from build123d import *

# Parameters (mm, degrees)
SKETCH2_R                           = 26
BOSS_EXTRUDE1_DEPTH                 = 110
CUT_EXTRUDE1_REACH                  = 117.983
CUT_EXTRUDE1_END_RADIUS             = 26
SKETCH3_W                           = 35
SKETCH3_H                           = 25
CUT_EXTRUDE1_DIRECTION_2_REACH      = 117.983
CUT_EXTRUDE1_DIRECTION_2_END_RADIUS = 26
CUT_EXTRUDE2_REACH                  = 118.211
CUT_EXTRUDE2_END_RADIUS             = 26
SKETCH4_R                           = 6
CUT_EXTRUDE4_REACH                  = 117.983
SKETCH6_W                           = 22
SKETCH6_H                           = 16
CUT_EXTRUDE4_DIRECTION_2_REACH      = 117.983


with BuildPart() as part:
    # Sketch2 → Boss-Extrude1 (new body)
    with BuildSketch(Plane(origin=(0, 0, 0), x_dir=(0, 0, -1), z_dir=(1, 0, 0))):
        Circle(SKETCH2_R)
    extrude(amount=BOSS_EXTRUDE1_DEPTH)

    # Cut-Extrude1: up to this cylinder (the profile starts inside it)
    cut_extrude1_end = Plane(origin=(54.2237205, 0, 0), z_dir=(-1, 0, 0)) * Cylinder(CUT_EXTRUDE1_END_RADIUS, 362.413441, mode=Mode.PRIVATE)
    # Sketch3 → Cut-Extrude1 (cut, up to the surface)
    with BuildSketch(Plane.XY, mode=Mode.PRIVATE) as cut_extrude1_sk1:
        with Locations((17.5, 13.5)):
            Rectangle(SKETCH3_W, SKETCH3_H)
    cut_extrude1_tool1 = extrude(cut_extrude1_sk1.sketch, amount=-CUT_EXTRUDE1_REACH, mode=Mode.PRIVATE) & cut_extrude1_end
    add(cut_extrude1_tool1.solids().sort_by_distance((17.5, 13.5, 0))[0], mode=Mode.SUBTRACT)
    # Sketch3 → Cut-Extrude1 (cut, up to the surface)
    with BuildSketch(Plane.XY, mode=Mode.PRIVATE) as cut_extrude1_sk2:
        Polygon((52.84232335, 26), (110, -7), (110, 26), align=None)
    cut_extrude1_tool2 = extrude(cut_extrude1_sk2.sketch, amount=-CUT_EXTRUDE1_REACH, mode=Mode.PRIVATE) & cut_extrude1_end
    add(cut_extrude1_tool2.solids().sort_by_distance((90.947441, 15, 0))[0], mode=Mode.SUBTRACT)

    # Cut-Extrude1 direction 2: up to this cylinder (the profile starts inside it)
    cut_extrude1_direction_2_end = Plane(origin=(54.2237205, 0, 0), z_dir=(-1, 0, 0)) * Cylinder(CUT_EXTRUDE1_DIRECTION_2_END_RADIUS, 362.413441, mode=Mode.PRIVATE)
    # Sketch3 → Cut-Extrude1 direction 2 (cut, up to the surface)
    with BuildSketch(Plane.XY, mode=Mode.PRIVATE) as cut_extrude1_direction_2_sk1:
        with Locations((17.5, 13.5)):
            Rectangle(SKETCH3_W, SKETCH3_H)
    cut_extrude1_direction_2_tool1 = extrude(cut_extrude1_direction_2_sk1.sketch, amount=CUT_EXTRUDE1_DIRECTION_2_REACH, mode=Mode.PRIVATE) & cut_extrude1_direction_2_end
    add(cut_extrude1_direction_2_tool1.solids().sort_by_distance((17.5, 13.5, 0))[0], mode=Mode.SUBTRACT)
    # Sketch3 → Cut-Extrude1 direction 2 (cut, up to the surface)
    with BuildSketch(Plane.XY, mode=Mode.PRIVATE) as cut_extrude1_direction_2_sk2:
        Polygon((52.84232335, 26), (110, -7), (110, 26), align=None)
    cut_extrude1_direction_2_tool2 = extrude(cut_extrude1_direction_2_sk2.sketch, amount=CUT_EXTRUDE1_DIRECTION_2_REACH, mode=Mode.PRIVATE) & cut_extrude1_direction_2_end
    add(cut_extrude1_direction_2_tool2.solids().sort_by_distance((90.947441, 15, 0))[0], mode=Mode.SUBTRACT)

    # Cut-Extrude2: up to this cylinder (the profile starts inside it)
    cut_extrude2_end = Plane(origin=(12, 0, 0), z_dir=(-1, 0, 0)) * Cylinder(CUT_EXTRUDE2_END_RADIUS, 289.422, mode=Mode.PRIVATE)
    # Sketch4 → Cut-Extrude2 (cut, up to the surface)
    with BuildSketch(Plane(origin=(0, 1, 0), x_dir=(1, 0, 0), z_dir=(0, 1, 0)), mode=Mode.PRIVATE) as cut_extrude2_sk1:
        with Locations(Location((12, 0, 0), (0, 0, 270))):
            Circle(SKETCH4_R)
    cut_extrude2_tool1 = extrude(cut_extrude2_sk1.sketch, amount=-CUT_EXTRUDE2_REACH, mode=Mode.PRIVATE) & cut_extrude2_end
    add(cut_extrude2_tool1.solids().sort_by_distance((12, 1, 0))[0], mode=Mode.SUBTRACT)

    # Sketch6 → Cut-Extrude4 (cut, up to next)
    with BuildSketch(Plane(origin=(0, 0, 0), x_dir=(1, 0, 0), z_dir=(0, 1, 0)), mode=Mode.PRIVATE) as cut_extrude4_sk1:
        with Locations((99, 18)):
            Rectangle(SKETCH6_W, SKETCH6_H)
    cut_extrude4_tool1 = extrude(cut_extrude4_sk1.sketch, amount=-CUT_EXTRUDE4_REACH, mode=Mode.PRIVATE) & part.part
    # Sketch6 → Cut-Extrude4 (cut, up to next)
    with BuildSketch(Plane(origin=(0, 0, 0), x_dir=(1, 0, 0), z_dir=(0, 1, 0)), mode=Mode.PRIVATE) as cut_extrude4_sk2:
        with Locations((99, -18)):
            Rectangle(SKETCH6_W, SKETCH6_H)
    cut_extrude4_tool2 = extrude(cut_extrude4_sk2.sketch, amount=-CUT_EXTRUDE4_REACH, mode=Mode.PRIVATE) & part.part
    add(cut_extrude4_tool1.solids().sort_by_distance((99, 0, -18))[0], mode=Mode.SUBTRACT)
    add(cut_extrude4_tool2.solids().sort_by_distance((99, 0, 18))[0], mode=Mode.SUBTRACT)

    # Sketch6 → Cut-Extrude4 direction 2 (cut, up to next)
    with BuildSketch(Plane(origin=(0, 0, 0), x_dir=(1, 0, 0), z_dir=(0, 1, 0)), mode=Mode.PRIVATE) as cut_extrude4_direction_2_sk1:
        with Locations((99, 18)):
            Rectangle(SKETCH6_W, SKETCH6_H)
    cut_extrude4_direction_2_tool1 = extrude(cut_extrude4_direction_2_sk1.sketch, amount=CUT_EXTRUDE4_DIRECTION_2_REACH, mode=Mode.PRIVATE) & part.part
    # Sketch6 → Cut-Extrude4 direction 2 (cut, up to next)
    with BuildSketch(Plane(origin=(0, 0, 0), x_dir=(1, 0, 0), z_dir=(0, 1, 0)), mode=Mode.PRIVATE) as cut_extrude4_direction_2_sk2:
        with Locations((99, -18)):
            Rectangle(SKETCH6_W, SKETCH6_H)
    cut_extrude4_direction_2_tool2 = extrude(cut_extrude4_direction_2_sk2.sketch, amount=CUT_EXTRUDE4_DIRECTION_2_REACH, mode=Mode.PRIVATE) & part.part
    add(cut_extrude4_direction_2_tool1.solids().sort_by_distance((99, 0, -18))[0], mode=Mode.SUBTRACT)
    add(cut_extrude4_direction_2_tool2.solids().sort_by_distance((99, 0, 18))[0], mode=Mode.SUBTRACT)


solid = part.part
Could you check a few things on this model? Use its own coordinates, in mm. A direction names the side the tool comes from. Give positions to 0.01 mm unless a question says otherwise; leave off trailing zeros. Order: outer loops, then holes, each group sorted by start corner. A loop starts at its lowest first (then second) coordinate and runs counter-clockwise, first axis right, second up.
1. I need wall thicknesses on L1, parallel to X at y = -8.25, z = 0; L2, parallel to X at y = -3, z = -11; L3, parallel to Z at x = 12, y = -19. Which ranges of each line are inside material? Lowest first, please.
Answers below:
L1: x = 0 to 6, 18 to 110
L2: x = 0 to 88
L3: z = -17.75 to -6, 6 to 17.75
2. Suppose I cut it at D-D (x = 25.5). Write out the boundary of the cut face in (y, z), plus the area to 3 significant figures.
Answers below:
outline: (1, -25.98) - (1, 25.98) arc R26 ccw (long way) to start
area: 1,110 mm2
3. Suppose I cut it at C-C (x = 12). Write out the boundary of the cut face in (y, z), plus the area to 3 significant figures.
Answers below:
outline: (-25.3, -6) arc R26 ccw to (1, -25.98) - (1, -6) - close; (-25.3, 6) - (1, 6) - (1, 25.98) arc R26 ccw to start
area: 793 mm2
4. Suppose I cut it at B-B (y = -21.5). Write out the boundary of the cut face in (x, z).
Answers below:
outline: (0, -14.62) - (88, -14.62) - (88, -10) - (110, -10) - (110, 10) - (88, 10) - (88, 14.62) - (0, 14.62) - close; hole circle Ø12 at (12, 0)
5. Which directions (+Z, -Z, +X, -X, +Y, -Y) give clear straight access to the entire face, cutting with the end or side of a thin tool? Please do faces 4 (the flat face through (88, -6, 16)), 5 (the flat face through (88, -6, -16)), 6 (the flat face through (110, -16, 0)).
Answers below:
face 4: +Z, +X, +Y, -Y
face 5: -Z, +X, +Y, -Y
face 6: +Z, -Z, +X, +Y, -Y
6. Thinking about a two-plate mould opening in X: for faces 1 (the flat face through (21, 1, 0)), 2 (the cylindrical face through (6.143, -12.316, -1.301)), 3 (the flat face through (35, 11, 0)), which applies, +X half, -X half, draft (parallel to the pull), parting line (faces both ways), or undercut?
Answers below:
face 1: draft
face 2: undercut
face 3: -X half
7. For pin 1 (12.5 mm diameter, centred on y = 10, z = -6, fed in from -X); pin 2 (1 mm diameter, centred on x = 14, z = -19.5, fed in from +Y); pin 3 (5 mm diameter, centred on y = -14.5, z = -20.5, fed in from +X); pin 4 (9.5 mm diameter, centred on x = 12, z = 0, fed in from -Y), each with a flat end and sliding along its axis, tell me the tip position at first contact or that it passes through.
Answers below:
pin 1: stops at x = 35
pin 2: stops at y = 1
pin 3: stops at x = 88
pin 4: passes through
8. Suppose I cut it at A-A (z = -13.5). Write out the boundary of the cut face in (x, y).
Answers below:
outline: (0, -22.22) - (88, -22.22) - (88, 5.7) - (59.39, 22.22) - (35, 22.22) - (35, 1) - (0, 1) - close
